Design review of the part built by this model. Coordinates are the model's own, in mm. A direction names the side the tool comes from. Give positions to 0.01 mm unless a question says otherwise; leave off trailing zeros. Write each loop counter-clockwise with the first axis right and the second up, starting at its lowest first coordinate (ties: lowest second). Pieces come first, ordered by that corner, then holes. Notation, with made-up numbers: (65.25, 18.25) -> (89.25, 18.25) arc R8 ccw to (89.25, 29.25) -> close; hole circle Ø9 at (51.5, 89). An arc over 180 degrees is marked (long way). Use CSV: the item, a comma, the result in double quotes.
```python
from build123d import *

# Parameters (mm, degrees)
F0_W      = 24
F0_H      = 5
F0_R      = 1.5
F0_R_2    = 0.4
F1_DEPTH  = 1
F2_W      = 24
F2_H      = 1
F3_DEPTH  = 15
F4_R      = 1.6
F5_DEPTH  = 25
F6_R      = 1.5
F7_W      = 1
F7_H      = 5
F8_DEPTH  = 1
F9_W      = 24
F9_H      = 1
F10_DEPTH = 2.5
F11_R     = 5
F12_R     = 2.5
F12_R_2   = 1.5
F13_DEPTH = 1.5
F14_R     = 2.5
F14_R_2   = 1.5
F15_DEPTH = 2
F16_R     = 3
F17_DEPTH = 25
F18_R     = 6


with BuildPart() as f1:
    # F0 (on Top) → F1 (new body)
    with BuildSketch(Plane.XY):
        Rectangle(F0_W, F0_H)
        with Locations((-7, 0)):
            Circle(F0_R, mode=Mode.SUBTRACT)
        with Locations((-2.49, 0)):
            Circle(F0_R_2, mode=Mode.SUBTRACT)
        with Locations((-0.83, 0)):
            Circle(F0_R_2, mode=Mode.SUBTRACT)
        with Locations((0.83, 0)):
            Circle(F0_R_2, mode=Mode.SUBTRACT)
        with Locations((2.49, 0)):
            Circle(F0_R_2, mode=Mode.SUBTRACT)
        with Locations((7, 0)):
            Circle(F0_R, mode=Mode.SUBTRACT)
    extrude(amount=F1_DEPTH)

    # F2 (on face) → F3 (join)
    with BuildSketch(Plane.XZ.offset(2.5)):
        with Locations((0, 0.5)):
            Rectangle(F2_W, F2_H)
    extrude(amount=F3_DEPTH)

    # F4 (on face) → F5 (cut)
    with BuildSketch(Plane(origin=(0, 0, 0), x_dir=(1, 0, 0), z_dir=(0, 0, -1))):
        with Locations((-7.75, 14)):
            Circle(F4_R)
        with Locations((7.75, 14)):
            Circle(F4_R)
    extrude(amount=-F5_DEPTH, mode=Mode.SUBTRACT)

    # F6
    f6_edges = [f1.edges().sort_by_distance(p)[0] for p in [
        (12, -17.5, 0.5),
        (-12, -17.5, 0.5),
    ]]
    fillet(f6_edges, radius=F6_R)

    # F7 (on face) → F8 (cut, through all)
    with BuildSketch(Plane(origin=(0, 0, 0), x_dir=(1, 0, 0), z_dir=(0, 0, -1))):
        with Locations((11.5, 10)):
            Rectangle(F7_W, F7_H)
        with Locations((-11.5, 10)):
            Rectangle(F7_W, F7_H)
    extrude(amount=-F8_DEPTH, mode=Mode.SUBTRACT)

    # F9 (on face) → F10 (join)
    with BuildSketch(Plane(origin=(0, 2.5, 0), x_dir=(-1, 0, 0), z_dir=(0, 1, 0))):
        with Locations((0, 0.5)):
            Rectangle(F9_W, F9_H)
    extrude(amount=F10_DEPTH)

    # F11
    f11_edges = [f1.edges().sort_by_distance(p)[0] for p in [
        (-12, 5, 0.5),
        (12, 5, 0.5),
    ]]
    fillet(f11_edges, radius=F11_R)

    # F12 (on face) → F13 (join)
    with BuildSketch(Plane(origin=(0, 0, 0), x_dir=(1, 0, 0), z_dir=(0, 0, -1))):
        with Locations((7, 0)):
            Circle(F12_R)
        with Locations((7, 0)):
            Circle(F12_R_2, mode=Mode.SUBTRACT)
        with Locations((-7, 0)):
            Circle(F12_R)
        with Locations((-7, 0)):
            Circle(F12_R_2, mode=Mode.SUBTRACT)
    extrude(amount=F13_DEPTH)

    # F14 (on face) → F15 (join)
    with BuildSketch(Plane.XY.offset(1)):
        with Locations((7, 0)):
            Circle(F14_R)
        with Locations((7, 0)):
            Circle(F14_R_2, mode=Mode.SUBTRACT)
        with Locations((-7, 0)):
            Circle(F14_R)
        with Locations((-7, 0)):
            Circle(F14_R_2, mode=Mode.SUBTRACT)
    extrude(amount=F15_DEPTH)

    # F16 (on face) → F17 (cut)
    with BuildSketch(Plane(origin=(0, 0, 0), x_dir=(1, 0, 0), z_dir=(0, 0, -1))):
        with Locations((0, -5)):
            Circle(F16_R)
    extrude(amount=-F17_DEPTH, mode=Mode.SUBTRACT)

    # F18
    f18_edges = [f1.edges().sort_by_distance(p)[0] for p in [
        (-3, 5, 0.5),
        (3, 5, 0.5),
    ]]
    fillet(f18_edges, radius=F18_R)


solid = f1.part
```
(1) Mouldability with a two-part tool opening along Y and no side actions: class faces 5 (the face through (9.385, -0.751, -0.74)), 6 (the face through (-11.5, -12.5, 0.5)), 7 (the face through (-7, 2, -1.5)) as +Y half, -Y half, draft (parallel to the pull), parting line (faces both ways), or undercut.
Established:
face 5,"parting line"
face 6,"undercut"
face 7,"draft"
(2) Tool access review of faces 1 (the face through (-11, -10, 0.5)), 2 (the face through (9.385, 0.751, 1.986)), 3 (the face through (11.5, -7.5, 0.5)), 4 (the face through (-4.29, 4.49, 0.49)): name each direction out of +Z, -Z, +X, -X, +Y, -Y from which nothing blocks a thin tool from reaching the whole face with its end or side.
Established:
face 1,"+Z, -Z, -X"
face 2,"+Z"
face 3,"+Z, -Z, +X"
face 4,"+Z, -Z, +Y"
(3) Take a section at C-C (x = -0.83). Write out the cut boundary in (y, z).
Established:
outline,"(-17.5, 0) -> (-0.4, 0) -> (-0.4, 1) -> (-17.5, 1) -> close; (0.4, 0) -> (2.12, 0) -> (2.12, 1) -> (0.4, 1) -> close"
(4) Clearance check with flat-ended pins moving along their axes: pin 1 (0.5 mm diameter, centred on x = -11.5, z = 0.5, fed in from -Y); pin 2 (3.5 mm diameter, centred on x = -7.75, y = -14, fed in from -Z); pin 3 (1 mm diameter, centred on y = -11, z = 0.5, fed in from +X); pin 4 (4 mm diameter, centred on x = 7, y = 0, fed in from -Z). State where each tip first meets the part, or that it passes through.
Established:
pin 1,"stops at y = -17.3"
pin 2,"stops at z = 0"
pin 3,"stops at x = 11"
pin 4,"stops at z = -1.5"
(5) Take a section at B-B (y = -14.75). Write out the cut boundary in (x, z).
Established:
outline,"(-12, 0) -> (-9.16, 0) -> (-9.16, 1) -> (-12, 1) -> close; (-6.34, 0) -> (6.34, 0) -> (6.34, 1) -> (-6.34, 1) -> close; (9.16, 0) -> (12, 0) -> (12, 1) -> (9.16, 1) -> close"
(6) Take a section at A-A (z = 1.8). Write out the cut boundary in (x, y), then the cut area to 3 significant figures.
Established:
outline,"circle Ø5 at (-7, 0); circle Ø5 at (7, 0); hole circle Ø3 at (-7, 0); hole circle Ø3 at (7, 0)"
area,"25.1 mm2"
(7) Take a section at D-D (x = -7.75). Write out the cut boundary in (y, z).
Established:
outline,"(-17.5, 0) -> (-15.6, 0) -> (-15.6, 1) -> (-17.5, 1) -> close; (-12.4, 0) -> (-2.38, 0) -> (-2.38, -1.5) -> (-1.3, -1.5) -> (-1.3, 3) -> (-2.38, 3) -> (-2.38, 1) -> (-12.4, 1) -> close; (1.3, -1.5) -> (2.38, -1.5) -> (2.38, 0) -> (4.94, 0) -> (4.94, 1) -> (2.38, 1) -> (2.38, 3) -> (1.3, 3) -> close"
(8) For line 1 along Y through (x, z) = (-8, 0.5); line 2 along Y through (x, z) = (7, 1.6); line 3 along X through (y, z) = (0.75, 0.85), list the stretches that pass through material, from the lowest coordinate up. Write a range as [from, to].
Established:
line 1,"y = [-17.5, -15.58], [-12.42, -1.12], [1.12, 4.9]"
line 2,"y = [-2.5, -1.5], [1.5, 2.5]"
line 3,"x = [-11.94, -8.3], [-5.7, 5.7], [8.3, 11.94]"
